from build123d import *

# Parameters (mm, degrees)
SKETCH1_W           = 315
SKETCH1_H           = 2
BOSS_EXTRUDE1_DEPTH = 200.5
SKETCH16_W          = 200.5
SKETCH16_H          = 2
BOSS_EXTRUDE2_DEPTH = 10
FILLET1_R           = 2
FILLET2_R           = 2
SKETCH17_R          = 2.5
CUT_EXTRUDE1_DEPTH  = 2
CUT_EXTRUDE2_DEPTH  = 2


with BuildPart() as part:
    # Sketch1 → Boss-Extrude1 (new body)
    with BuildSketch(Plane(origin=(0, 0, 0), x_dir=(0, 0, -1), z_dir=(1, 0, 0))):
        with Locations((157.5, 1)):
            Rectangle(SKETCH1_W, SKETCH1_H)
    extrude(amount=BOSS_EXTRUDE1_DEPTH)

    # Sketch16 → Boss-Extrude2 (add)
    with BuildSketch(Plane.XZ):
        with Locations((100.25, -314)):
            Rectangle(SKETCH16_W, SKETCH16_H)
    extrude(amount=BOSS_EXTRUDE2_DEPTH)

    # Fillet1
    fillet1_edges = [part.edges().sort_by_distance(p)[0] for p in [
        (100.25, 2, -315),
    ]]
    fillet(fillet1_edges, radius=FILLET1_R)

    # Fillet2
    fillet2_edges = [part.edges().sort_by_distance(p)[0] for p in [
        (100.25, 0, -313),
    ]]
    fillet(fillet2_edges, radius=FILLET2_R)

    # Sketch17 → Cut-Extrude1 (cut)
    with BuildSketch(Plane(origin=(0, 0, -315), x_dir=(-1, 0, 0), z_dir=(0, 0, -1))):
        with Locations((-193, -5)):
            Circle(SKETCH17_R)
        with Locations((-7.5, -5)):
            Circle(SKETCH17_R)
    extrude(amount=-CUT_EXTRUDE1_DEPTH, mode=Mode.SUBTRACT)

    # Sketch19 → Cut-Extrude2 (cut)
    with BuildSketch(Plane(origin=(0, 2, 0), x_dir=(1, 0, 0), z_dir=(0, 1, 0))):
        with BuildLine():
            Line((163.5, 20.25), (163.5, 7.75))
            ThreePointArc((163.5, 7.75), (166, 5.25), (168.5, 7.75))
            Line((168.5, 7.75), (168.5, 20.25))
            ThreePointArc((168.5, 20.25), (166, 22.75), (163.5, 20.25))
        make_face()
    extrude(amount=-CUT_EXTRUDE2_DEPTH, mode=Mode.SUBTRACT)


solid = part.part
Verification items for the finished model (mm, model axes). A direction names the side the tool comes from. Coordinates: 2 decimals unless noted, no trailing zeros. Order: outer loops, then holes, each group sorted by start corner. A loop starts at its lowest first (then second) coordinate and runs counter-clockwise, first axis right, second up.
1. Scan lines: line 1 (Z direction, x = 15.5, y = -2.5); line 2 (Y direction, x = 7.5, z = -314.2); line 3 (Y direction, x = 193, z = -313.75). Record each from-to range of solid material in increasing order.
Results found:
line 1: z = -315 to -313
line 2: y = -10 to -7.5, -2.5 to 1.6
line 3: y = -10 to -7.5, -2.5 to 1.85
2. Sectioned sample at A-A, the plane y = -5. Record the cut outline in (x, z), and give its area (3 significant figures).
Results found:
outline: (0, -315) - (5, -315) - (5, -313) - (0, -313) - close; (10, -315) - (190.5, -315) - (190.5, -313) - (10, -313) - close; (195.5, -315) - (200.5, -315) - (200.5, -313) - (195.5, -313) - close
area: 381 mm2
3. Go/stop test with flat-tipped pins: pin 1 Ø0.6 at (y, z) = (1, -14) entering from -X; pin 2 Ø1.5 at (x, z) = (159.5, -197) entering from -Y; pin 3 Ø6.5 at (x, y) = (116, -6.5) entering from +Z; pin 4 Ø4 at (x, y) = (7.5, -5) entering from -Z. Record where each tip stops, or that it passes through.
Results found:
pin 1: stops at x = 0
pin 2: stops at y = 0
pin 3: stops at z = -313
pin 4: passes through
4. Sectioned sample at B-B, the plane x = 141.5. Record the cut outline in (y, z).
Results found:
outline: (-10, -315) - (0, -315) arc R2 ccw to (2, -313) - (2, 0) - (0, 0) - (0, -311) arc R2 cw to (-2, -313) - (-10, -313) - close
5. Sectioned sample at C-C, the plane z = -182.5. Record the cut outline in (x, y), and give its area (3 significant figures).
Results found:
outline: (0, 0) - (200.5, 0) - (200.5, 2) - (0, 2) - close
area: 401 mm2
6. Set-up check for faces 1 (the face through (200.5, 1, -158)), 2 (the face through (99, -6, -313)): record each of +Z, -Z, +X, -X, +Y, -Y from which the full face is reachable in a straight line by a thin tool's end or side.
Results found:
face 1: +Z, -Z, +X, +Y, -Y
face 2: +Z, +X, -X, -Y
